Design review of the part built by this model. Coordinates are the model's own, in mm. A direction names the side the tool comes from. Round coordinates to 2 decimals unless told otherwise and drop trailing zeros. Write each question's results on one line, items separated by ' | '. Start each with the question number.
from build123d import *

# Parameters (mm, degrees)
SKETCH1_W           = 150
SKETCH1_H           = 140
BOSS_EXTRUDE1_DEPTH = 85
SKETCH2_W           = 31.205424041
SKETCH2_H           = 21.045678937
CUT_EXTRUDE1_DEPTH  = 1
SKETCH3_W           = 95.813101978
SKETCH3_H           = 125.386699306
CUT_EXTRUDE2_DEPTH  = 1


with BuildPart() as part:
    # Sketch1 → Boss-Extrude1 (new body)
    with BuildSketch(Plane(origin=(0, 0, 0), x_dir=(1, 0, 0), z_dir=(0, 1, 0))):
        Rectangle(SKETCH1_W, SKETCH1_H)
    extrude(amount=BOSS_EXTRUDE1_DEPTH)

    # Sketch2 → Cut-Extrude1 (cut)
    with BuildSketch(Plane.XY.offset(70)):
        with Locations((47.705903702, 18.235389002)):
            Rectangle(SKETCH2_W, SKETCH2_H)
    extrude(amount=-CUT_EXTRUDE1_DEPTH, mode=Mode.SUBTRACT)

    # Sketch3 → Cut-Extrude2 (cut)
    with BuildSketch(Plane(origin=(0, 85, 0), x_dir=(1, 0, 0), z_dir=(0, 1, 0))):
        with Locations((-19.67334308, 0)):
            Rectangle(SKETCH3_W, SKETCH3_H)
    extrude(amount=-CUT_EXTRUDE2_DEPTH, mode=Mode.SUBTRACT)


solid = part.part
1) To check wall thickness, follow line 1 (Y direction, x = 26.5, z = 30.5); line 2 (Z direction, x = 61.5, y = 19.5). State the ranges of each line that lie inside material, in increasing order. Write a range as from..to.
2) For faces 1 (the face through (-75, 42, 1)), 2 (the face through (47, 18, 69)), list the 3-axis set-ups (+Z, -Z, +X, -X, +Y, -Y) from which the entire face can be reached by the end or side of a thin tool; tool diameter is ignored.
3) The part is to be moulded in two halves that separate along Z. For faces 3 (the face through (-20, 84, -1)), 4 (the face through (75, 42, 1)), 5 (the face through (-1, 42, -70)), say which applies: +Z half, -Z half, draft (parallel to the pull), parting line (faces both ways), or undercut.
Geometry check:
1) line 1: y = 0..84 | line 2: z = -70..69
2) face 1: +Z, -Z, -X, +Y, -Y | face 2: +Z
3) face 3: undercut | face 4: draft | face 5: -Z half
